Source: CAD feature listing. Evaluate the final solid. Frame: model axes, mm. Face numbers are marked on the shaded views. A direction names the side the tool comes from. Round coordinates to 2 decimals unless told otherwise and drop trailing zeros. Write each loop counter-clockwise with the first axis right and the second up, starting at its lowest first coordinate (ties: lowest second). Pieces come first, ordered by that corner, then holes.
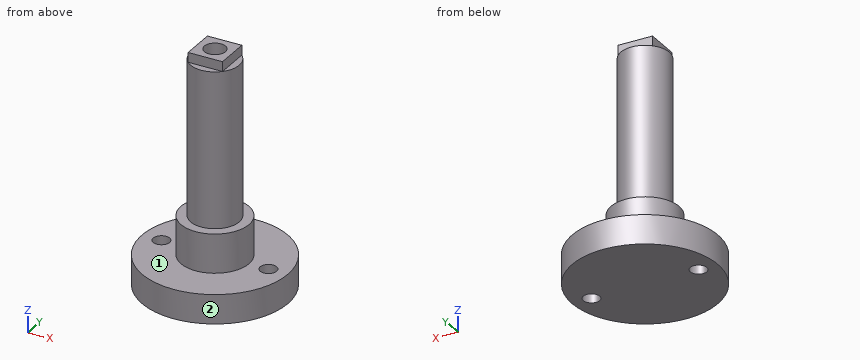
from build123d import *

# Parameters (mm, degrees)
F0_R     = 3.96875
F1_DEPTH = 25.4
F2_W     = 5.61266
F2_H     = 5.61266
F3_DEPTH = 1.5875
F4_R     = 1.7272
F5_DEPTH = 6.35
F6_R     = 5.55625
F7_DEPTH = 6.35
F8_R     = 11.90625
F8_R_2   = 1.35255
F9_DEPTH = 4.7625


with BuildPart() as f1:
    # F0 (on Top) → F1 (new body)
    with BuildSketch(Plane.XY):
        Circle(F0_R)
    extrude(amount=F1_DEPTH)

    # F2 (on face) → F3 (join)
    with BuildSketch(Plane.XY.offset(25.4)):
        Rectangle(F2_W, F2_H)
    extrude(amount=F3_DEPTH)

    # F4 (on face) → F5 (cut)
    with BuildSketch(Plane.XY.offset(26.9875)):
        Circle(F4_R)
    extrude(amount=-F5_DEPTH, mode=Mode.SUBTRACT)

    # F6 (on face) → F7 (join)
    with BuildSketch(Plane(origin=(0, 0, 0), x_dir=(1, 0, 0), z_dir=(0, 0, -1))):
        Circle(F6_R)
    extrude(amount=F7_DEPTH)

    # F8 (on face) → F9 (join)
    with BuildSketch(Plane(origin=(0, 0, -6.35), x_dir=(1, 0, 0), z_dir=(0, 0, -1))):
        Circle(F8_R)
        with Locations((-8.73125, 0)):
            Circle(F8_R_2, mode=Mode.SUBTRACT)
        with Locations((8.73125, 0)):
            Circle(F8_R_2, mode=Mode.SUBTRACT)
    extrude(amount=F9_DEPTH)


solid = f1.part
1) Section query C-C on z = 1.5. Return the cut outline in (x, y).
Taken from the geometry:
outline: circle Ø7.94 at (0, 0)
2) Reachability of the marked faces 1 and 2 from +Z, -Z, +X, -X, +Y, -Y: full face, straight path, thin tool, end or side. Return the list, or none.
Taken from the geometry:
face 1: +Z
face 2: +Z, -Z
3) Contact query for flat-ended pins moving along their axis: P1, Ø1, axis at x = -8.5, y = -5, coming from the +Z side; P2, Ø6, axis at y = -7.5, z = -1.5, coming from the +X side; P3, Ø4, axis at y = 3.5, z = 12, coming from the +X side. Output: stop coordinate, or through.
Taken from the geometry:
P1: stops at z = -6.35
P2: stops at x = 3.26
P3: stops at x = 3.67
4) Section query B-B on x = 0. Return the cut outline in (y, z), then the cut area to 3 significant figures.
Taken from the geometry:
outline: (-11.91, -11.11) - (11.91, -11.11) - (11.91, -6.35) - (5.56, -6.35) - (5.56, 0) - (3.97, 0) - (3.97, 25.4) - (2.81, 25.4) - (2.81, 26.99) - (1.73, 26.99) - (1.73, 20.64) - (-1.73, 20.64) - (-1.73, 26.99) - (-2.81, 26.99) - (-2.81, 25.4) - (-3.97, 25.4) - (-3.97, 0) - (-5.56, 0) - (-5.56, -6.35) - (-11.91, -6.35) - close
area: 373 mm2
5) Material intervals for line 1 (X direction, y = 0, z = -9.05); line 2 (Y direction, x = 0, z = 23.75); line 3 (Z direction, x = -4.25, y = -4.25), sorted ascending.
Taken from the geometry:
line 1: x = -11.91 to -10.08, -7.38 to 7.38, 10.08 to 11.91
line 2: y = -3.97 to -1.73, 1.73 to 3.97
line 3: z = -11.11 to -6.35
6) Section query D-D on y = 4.5. Return the cut outline in (x, z), then the cut area to 3 significant figures.
Taken from the geometry:
outline: (-11.02, -11.11) - (11.02, -11.11) - (11.02, -6.35) - (3.26, -6.35) - (3.26, 0) - (-3.26, 0) - (-3.26, -6.35) - (-11.02, -6.35) - close
area: 146 mm2
7) Section query A-A on y = 0. Return the cut outline in (x, z).
Taken from the geometry:
outline: (-11.91, -11.11) - (-10.08, -11.11) - (-10.08, -6.35) - (-11.91, -6.35) - close; (-7.38, -11.11) - (7.38, -11.11) - (7.38, -6.35) - (5.56, -6.35) - (5.56, 0) - (3.97, 0) - (3.97, 25.4) - (2.81, 25.4) - (2.81, 26.99) - (1.73, 26.99) - (1.73, 20.64) - (-1.73, 20.64) - (-1.73, 26.99) - (-2.81, 26.99) - (-2.81, 25.4) - (-3.97, 25.4) - (-3.97, 0) - (-5.56, 0) - (-5.56, -6.35) - (-7.38, -6.35) - close; (10.08, -11.11) - (11.91, -11.11) - (11.91, -6.35) - (10.08, -6.35) - close
